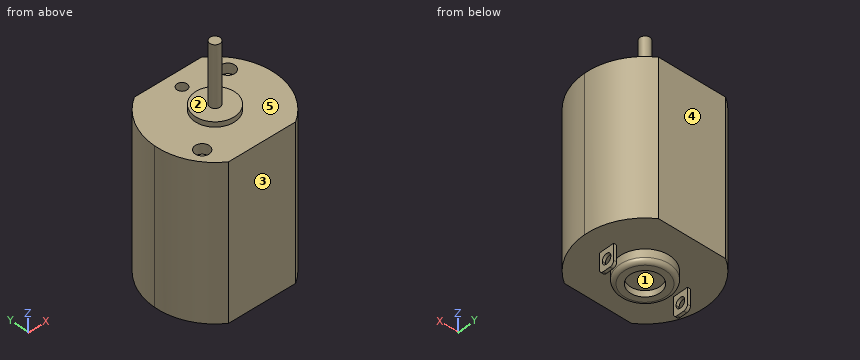
from build123d import *

# Parameters (mm, degrees)
SKETCH_1_W          = 0.3
SKETCH_1_H          = 1.5
SKETCH_1_R          = 2.5
SKETCH_1_R_2        = 1.5
EXTRUDE_1_DEPTH     = 15.2
SKETCH_1_4_W        = 0.3
SKETCH_1_4_H        = 1.5
EXTRUDE_2_DEPTH     = 2
CUT_EXTRUDE_2_DEPTH = 19.763794925
FILLET_1_R          = 0.4
SKETCH_1_5_R        = 2.5
SKETCH_1_5_R_2      = 1.5
EXTRUDE_3_DEPTH     = 1.2
CUT_EXTRUDE_START   = -1.2
SKETCH_1_7_R        = 1.5
CUT_EXTRUDE_1_DEPTH = 0.6
FILLET_2_R          = 0.4
SKETCH_3_R          = 2
EXTRUDE_4_DEPTH     = 0.5
SKETCH_3_3_R        = 0.5
EXTRUDE_5_DEPTH     = 6.5
SKETCH_4_R          = 0.7
SKETCH_4_R_2        = 0.5
CUT_EXTRUDE_3_DEPTH = 1


with BuildPart() as part:
    # 草图1 → 凸台-拉伸1 (new body)
    # profile 1 of 5: a face of its own
    with BuildSketch(Plane.XY):
        with BuildLine():
            ThreePointArc((-6, 0), (-5.286764074, -2.837274331), (-3.31662479, -5))
            Line((-3.31662479, -5), (3.31662479, -5))
            ThreePointArc((3.31662479, -5), (5.286764074, -2.837274331), (6, 0))
            ThreePointArc((6, 0), (5.286764074, 2.837274331), (3.31662479, 5))
            Line((3.31662479, 5), (-3.31662479, 5))
            ThreePointArc((-3.31662479, 5), (-5.286764074, 2.837274331), (-6, 0))
        make_face()
        with Locations((-3.65, 0)):
            Rectangle(SKETCH_1_W, SKETCH_1_H, mode=Mode.SUBTRACT)
        Circle(SKETCH_1_R, mode=Mode.SUBTRACT)
        with Locations((3.65, 0)):
            Rectangle(SKETCH_1_W, SKETCH_1_H, mode=Mode.SUBTRACT)
    # profile 2 of 5: a face of its own
    with BuildSketch(Plane.XY):
        Circle(SKETCH_1_R)
        Circle(SKETCH_1_R_2, mode=Mode.SUBTRACT)
    # profile 3 of 5: a face of its own
    with BuildSketch(Plane.XY):
        Circle(SKETCH_1_R_2)
    # profile 4 of 5: a face of its own
    with BuildSketch(Plane.XY):
        with Locations((3.65, 0)):
            Rectangle(SKETCH_1_W, SKETCH_1_H)
    # profile 5 of 5: a face of its own
    with BuildSketch(Plane.XY):
        with Locations((-3.65, 0)):
            Rectangle(SKETCH_1_W, SKETCH_1_H)
    extrude(amount=EXTRUDE_1_DEPTH)

    # 草图1<4> → 凸台-拉伸2 (add)
    with BuildSketch(Plane.XY):
        with Locations((3.65, 0)):
            Rectangle(SKETCH_1_4_W, SKETCH_1_4_H)
        with Locations((-3.65, 0)):
            Rectangle(SKETCH_1_4_W, SKETCH_1_4_H)
    extrude(amount=-EXTRUDE_2_DEPTH)

    # 草图2 → 切除-拉伸2 (cut, through all)
    with BuildSketch(Plane(origin=(3.8, 0, 0), x_dir=(0, 0, -1), z_dir=(1, 0, 0))):
        with BuildLine():
            Line((0.95, 0.45), (1.05, 0.45))
            ThreePointArc((1.05, 0.45), (1.5, 0), (1.05, -0.45))
            Line((1.05, -0.45), (0.95, -0.45))
            ThreePointArc((0.95, -0.45), (0.5, 0), (0.95, 0.45))
        make_face()
    extrude(amount=-CUT_EXTRUDE_2_DEPTH, mode=Mode.SUBTRACT)

    # 圆角1
    fillet_1_edges = [part.edges().sort_by_distance(p)[0] for p in [
        (3.65, -0.75, -2),
        (3.65, 0.75, -2),
        (-3.65, -0.75, -2),
        (-3.65, 0.75, -2),
    ]]
    fillet(fillet_1_edges, radius=FILLET_1_R)

    # 草图1<5> → 凸台-拉伸3 (add)
    # profile 1 of 2: a face of its own
    with BuildSketch(Plane.XY):
        Circle(SKETCH_1_5_R)
        Circle(SKETCH_1_5_R_2, mode=Mode.SUBTRACT)
    # profile 2 of 2: a face of its own
    with BuildSketch(Plane.XY):
        Circle(SKETCH_1_5_R_2)
    extrude(amount=-EXTRUDE_3_DEPTH)

    # 草图1<7> → 切除-拉伸1 (cut)
    with BuildSketch(Plane.XY.offset(CUT_EXTRUDE_START)):
        Circle(SKETCH_1_7_R)
    extrude(amount=CUT_EXTRUDE_1_DEPTH, mode=Mode.SUBTRACT)

    # 圆角2
    fillet_2_edges = [part.edges().sort_by_distance(p)[0] for p in [
        (-2.5, 0, -1.2),
    ]]
    fillet(fillet_2_edges, radius=FILLET_2_R)

    # 草图3 → 凸台-拉伸4 (add)
    with BuildSketch(Plane.XY.offset(15.2)):
        Circle(SKETCH_3_R)
    extrude(amount=EXTRUDE_4_DEPTH)

    # 草图3<3> → 凸台-拉伸5 (add)
    with BuildSketch(Plane.XY.offset(15.2)):
        Circle(SKETCH_3_3_R)
    extrude(amount=EXTRUDE_5_DEPTH)

    # 草图4 → 切除-拉伸3 (cut)
    with BuildSketch(Plane.XY.offset(15.2)):
        with Locations((-3.785828839, -2.7)):
            Circle(SKETCH_4_R)
        with Locations((3.785828839, 2.7)):
            Circle(SKETCH_4_R)
        with Locations((0, 3.5)):
            Circle(SKETCH_4_R_2)
    extrude(amount=-CUT_EXTRUDE_3_DEPTH, mode=Mode.SUBTRACT)


solid = part.part
The listing builds one solid part. Answer for the finished solid, in the listing's coordinates (mm). Face numbers are marked on the shaded views. A direction names the side the tool comes from. Round coordinates to 2 decimals unless told otherwise and drop trailing zeros. Write each loop counter-clockwise with the first axis right and the second up, starting at its lowest first coordinate (ties: lowest second). Pieces come first, ordered by that corner, then holes. Notation, with made-up numbers: (64.5, 83.25) - (81.5, 83.25) arc R22 cw to (81.5, 103.25) - close; hole circle Ø9 at (28.25, 83.25). An arc over 180 degrees is marked (long way). Use a Markdown table: item, result. Add a question column.
1. The part is cut by section C-C (x = -5). Write down the section's boundary in (y, z), and give its area (3 significant figures).
2. Consider line 1 (Y direction, x = 0, z = 14.6); line 2 (Z direction, x = -1.5, y = -1); line 3 (Z direction, x = -3.75, y = -3). Determine where each line is inside the solid, lowest interval first.
3. The part is cut by section A-A (x = 0). Write down the section's boundary in (y, z), and give its area (3 significant figures).
4. The part is cut by section D-D (z = 8). Write down the section's boundary in (x, y).
5. A tool of negligible diameter and unlimited length cuts with its end or side. For the marked faces 4 and 5, from which of +Z, -Z, +X, -X, +Y, -Y can it reach the whole face along a straight path? Write none if from no direction.
6. The part is cut by section B-B (z = 17.75). Write down the section's boundary in (x, y).
7. Flat-ended cylindrical pins translate along their axes: P1, Ø1.6, axis at x = 3.79, y = 2.7, coming from the +Z side; P2, Ø2, axis at y = -3.5, z = 8, coming from the +X side; P3, Ø3, axis at y = -4, z = 18.5, coming from the +X side; P4, Ø4, axis at y = 4, z = 12, coming from the -X side. Find the tip coordinate at first contact, or state that the pin passes through.
8. For a pull along Y with two mould halves and no side action, classify the marked faces 1, 2 and 3 as +Y half, -Y half, draft (parallel to the pull), parting line (faces both ways), or undercut.
Reported:
| question | item | result |
|---|---|---|
| 1 | outline | (-3.32, 0) - (3.32, 0) - (3.32, 15.2) - (-3.32, 15.2) - close |
| 1 | area | 101 mm^2 |
| 2 | line 1 | -5 to 3, 4 to 5 |
| 2 | line 2 | -1.2 to 15.7 |
| 2 | line 3 | 0 to 14.2 |
| 3 | outline | (-5, 0) - (-2.5, 0) - (-2.5, -0.8) arc R0.4 ccw to (-2.1, -1.2) - (-1.5, -1.2) - (-1.5, -0.6) - (1.5, -0.6) - (1.5, -1.2) - (2.1, -1.2) arc R0.4 ccw to (2.5, -0.8) - (2.5, 0) - (5, 0) - (5, 15.2) - (4, 15.2) - (4, 14.2) - (3, 14.2) - (3, 15.2) - (2, 15.2) - (2, 15.7) - (0.5, 15.7) - (0.5, 21.7) - (-0.5, 21.7) - (-0.5, 15.7) - (-2, 15.7) - (-2, 15.2) - (-5, 15.2) - close |
| 3 | area | 163 mm^2 |
| 4 | outline | (-3.32, -5) - (3.32, -5) arc R6 ccw to (3.32, 5) - (-3.32, 5) arc R6 ccw to start |
| 5 | face 4 | +Z, -Z, +X, -X, +Y |
| 5 | face 5 | +Z |
| 6 | outline | circle Ø1 at (0, 0) |
| 7 | P1 | z = 15.2 |
| 7 | P2 | x = 5.45 |
| 7 | P3 | through |
| 7 | P4 | x = -5.66 |
| 8 | face 1 | undercut |
| 8 | face 2 | draft |
| 8 | face 3 | -Y half |
